from build123d import *

# Parameters (mm, degrees)
SKETCH1_W           = 155.702807198
SKETCH1_H           = 58
SKETCH1_R           = 1.5
BOSS_EXTRUDE2_DEPTH = 2
SKETCH2_W           = 5
SKETCH2_H           = 88
BOSS_EXTRUDE3_DEPTH = 2
SKETCH3_R           = 11.15
CUT_EXTRUDE1_DEPTH  = 10
SKETCH4_R           = 1.5
BOSS_EXTRUDE4_DEPTH = 2
SKETCH7_W           = 1.5
SKETCH7_H           = 88
SKETCH7_H_2         = 87.852132556
CUT_EXTRUDE2_DEPTH  = 10
SKETCH8_W           = 0.36402546
SKETCH8_H           = 0.147867444
SKETCH8_W_2         = 1.5
SKETCH8_W_3         = 1
SKETCH8_H_2         = 88
CUT_EXTRUDE5_DEPTH  = 66.5


with BuildPart() as part:
    # Sketch1 → Boss-Extrude2 (new body)
    with BuildSketch(Plane(origin=(0, 0, 0), x_dir=(1, 0, 0), z_dir=(0, 1, 0))):
        with Locations((1.171695753, -5)):
            Rectangle(SKETCH1_W, SKETCH1_H)
        Polygon((-76.679707846, 44), (-76.679707846, 24), (79.023099352, 24), (79.023099352, 44), (62.885457038, 44), (59.885457038, 44), (-57.542065533, 44), (-60.542065533, 44), align=None)
        with Locations((-59.042065533, 34)):
            Circle(SKETCH1_R, mode=Mode.SUBTRACT)
        with Locations((61.385457038, 34)):
            Circle(SKETCH1_R, mode=Mode.SUBTRACT)
        Polygon((-76.679707846, -44), (-60.542065533, -44), (-57.542065533, -44), (59.885457038, -44), (62.885457038, -44), (79.023099352, -44), (79.023099352, -34), (-76.679707846, -34), align=None)
        with Locations((-59.042065533, -39)):
            Circle(SKETCH1_R, mode=Mode.SUBTRACT)
        with Locations((61.385457038, -39)):
            Circle(SKETCH1_R, mode=Mode.SUBTRACT)
    extrude(amount=BOSS_EXTRUDE2_DEPTH)

    # Sketch2 → Boss-Extrude3 (add)
    with BuildSketch(Plane(origin=(0, 2, 0), x_dir=(1, 0, 0), z_dir=(0, 1, 0))):
        with Locations((81.523099352, 0)):
            Rectangle(SKETCH2_W, SKETCH2_H)
        with Locations((-79.179707846, 0)):
            Rectangle(SKETCH2_W, SKETCH2_H)
    extrude(amount=-BOSS_EXTRUDE3_DEPTH)

    # Sketch3 → Cut-Extrude1 (cut)
    with BuildSketch(Plane(origin=(0, 2, 0), x_dir=(1, 0, 0), z_dir=(0, 1, 0))):
        with Locations((-28.93518489, -2.5)):
            Circle(SKETCH3_R)
        with Locations((31.278576395, -2.5)):
            Circle(SKETCH3_R)
    extrude(amount=-CUT_EXTRUDE1_DEPTH, mode=Mode.SUBTRACT)

    # Sketch4 → Boss-Extrude4 (add)
    with BuildSketch(Plane(origin=(0, 2, 0), x_dir=(1, 0, 0), z_dir=(0, 1, 0))):
        Polygon((-23.828304247, 44), (26.171695753, 44), (26.171695753, 50.823606938), (13.671695753, 56.49492606), (-11.328304247, 56.49492606), (-23.828304247, 50.823606938), align=None)
        with Locations((1.171695753, 50.24746303)):
            Circle(SKETCH4_R, mode=Mode.SUBTRACT)
    extrude(amount=-BOSS_EXTRUDE4_DEPTH)

    # Sketch7 → Cut-Extrude2 (cut)
    with BuildSketch(Plane(origin=(0, 2, 0), x_dir=(1, 0, 0), z_dir=(0, 1, 0))):
        with Locations((-80.929707846, 0)):
            Rectangle(SKETCH7_W, SKETCH7_H)
        with Locations((83.273099352, 0.073933722)):
            Rectangle(SKETCH7_W, SKETCH7_H_2)
    extrude(amount=-CUT_EXTRUDE2_DEPTH, mode=Mode.SUBTRACT)

    # Sketch8 → Cut-Extrude5 (cut)
    with BuildSketch(Plane(origin=(0, 2, 0), x_dir=(1, 0, 0), z_dir=(0, 1, 0))):
        with Locations((82.341086622, -43.926066278)):
            Rectangle(SKETCH8_W, SKETCH8_H)
        with Locations((83.273099352, -43.926066278)):
            Rectangle(SKETCH8_W_2, SKETCH8_H)
        Polygon((81.523099352, 44), (81.523099352, -44), (82.159073892, -44), (82.159073892, -43.852132556), (82.523099352, -43.852132556), (82.523099352, 44), align=None)
        with Locations((-79.679707846, 0)):
            Rectangle(SKETCH8_W_3, SKETCH8_H_2)
    extrude(amount=-CUT_EXTRUDE5_DEPTH, mode=Mode.SUBTRACT)


solid = part.part
Could you check a few things on this model? Use its own coordinates, in mm. Round coordinates to 2 decimals unless told otherwise and drop trailing zeros. Order: outer loops, then holes, each group sorted by start corner. A loop starts at its lowest first (then second) coordinate and runs counter-clockwise, first axis right, second up.
Q1. Imagine slicing it at C-C, the plane x = -68.5. List the corners of the cut face in (y, z) for me.
Geometry says:
outline: (0, -44) - (2, -44) - (2, 44) - (0, 44) - close
Q2. Imagine slicing it at A-A, the plane z = 2.5. List the corners of the cut face in (x, y) for me.
Geometry says:
outline: (-79.18, 0) - (-40.09, 0) - (-40.09, 2) - (-79.18, 2) - close; (-17.79, 0) - (20.13, 0) - (20.13, 2) - (-17.79, 2) - close; (42.43, 0) - (81.52, 0) - (81.52, 2) - (42.43, 2) - close
Q3. Thinking about a two-plate mould opening in Z: for faces 1 (the face through (0.847, 1.014, -48.783)), 2 (the face through (20.01, 1.01, -53.62)), 3 (the face through (0, 2, -7)), 4 (the face through (-40.074, 1.014, 2.01)), which applies, released by +Z, released by -Z, zero draft, split by the parting line, or undercut?
Geometry says:
face 1: undercut
face 2: released by -Z
face 3: zero draft
face 4: undercut
Q4. I'm going to push flat-ended pins straight in: P1, Ø1, axis at y = 1, z = -48, coming from the -X side; P2, Ø0.6, axis at y = 1.5, z = -48.5, coming from the +X side. Where does each tip first touch, or does it pass through?
Geometry says:
P1: stops at x = -23.83
P2: stops at x = 26.17
Q5. Imagine slicing it at B-B, the plane y = 0.5. List the corners of the cut face in (x, z) for me, then the cut area to 3 significant figures.
Geometry says:
outline: (-79.18, -44) - (-23.83, -44) - (-23.83, -50.82) - (-11.33, -56.49) - (13.67, -56.49) - (26.17, -50.82) - (26.17, -44) - (81.52, -44) - (81.52, 44) - (-79.18, 44) - close; hole circle Ø3 at (-59.04, -34); hole circle Ø3 at (-59.04, 39); hole circle Ø22.3 at (-28.94, 2.5); hole circle Ø3 at (1.17, -50.25); hole circle Ø22.3 at (31.28, 2.5); hole circle Ø3 at (61.39, -34); hole circle Ø3 at (61.39, 39)
area: 13,900 mm2
Q6. Please list where these lines run through material, in increasing order: probe 1 along X at (y, z) = (0.9, 2.5); probe 2 along X at (y, z) = (1, 39); probe 3 along Z at (x, y) = (1, 1.85).
Geometry says:
probe 1: x = -79.18 to -40.09, -17.79 to 20.13, 42.43 to 81.52
probe 2: x = -79.18 to -60.54, -57.54 to 59.89, 62.89 to 81.52
probe 3: z = -56.49 to -51.74, -48.76 to 44
